Could you check a few things on this drawing? It's one solid part, dimensions in mm from its lowest x, y, z. A direction names the side the tool comes from. Give positions to 0.01 mm unless a question says otherwise; leave off trailing zeros. Loops run counter-clockwise (first coordinate to the right, second up) from the corner with the lowest first, then second, coordinate; pieces in that order, holes last. Notation, with made-up numbers: M 47,73.25 L 54,73.25 A18 ccw 54,84.25 Z; hole C -40,46.25 d5. An arc over 180 degrees is marked long. Answer as CSV lines item,"result". Start each with the question number.
Item 1: I want a section at C-C on y = 20. List the corners of the cut face in (x, z) for me (1 decimal).
Item 2: I want a section at A-A on x = 15.24. List the corners of the cut face in (y, z) for me (1 decimal).
Item 3: I want a section at B-B on x = 22. List the corners of the cut face in (y, z) for me (1 decimal).
Item 4: If we mould it in two halves opening along X, with no side actions, what happens to the marked faces 1, 2, 3 and 4? For each: released by +X, released by -X, zero draft, split by the parting line, or undercut.
Item 5: I want a section at D-D on z = 5.5. List the corners of the cut face in (x, y) for me.
Item 6: For the marked faces 5 and 6, which set-ups out of +Z, -Z, +X, -X, +Y, -Y let a thin tool reach every point of the face, with its end or its side?
Item 7: If I drill on line 1 along X through (y, z) = (14, 20); line 2 along Y through (x, z) = (5, 11.75); line 3 along X through (y, z) = (24.25, 13.5) (1 decimal), over which ranges is the centre line in solid material (lowest first)? Write a range as from..to.
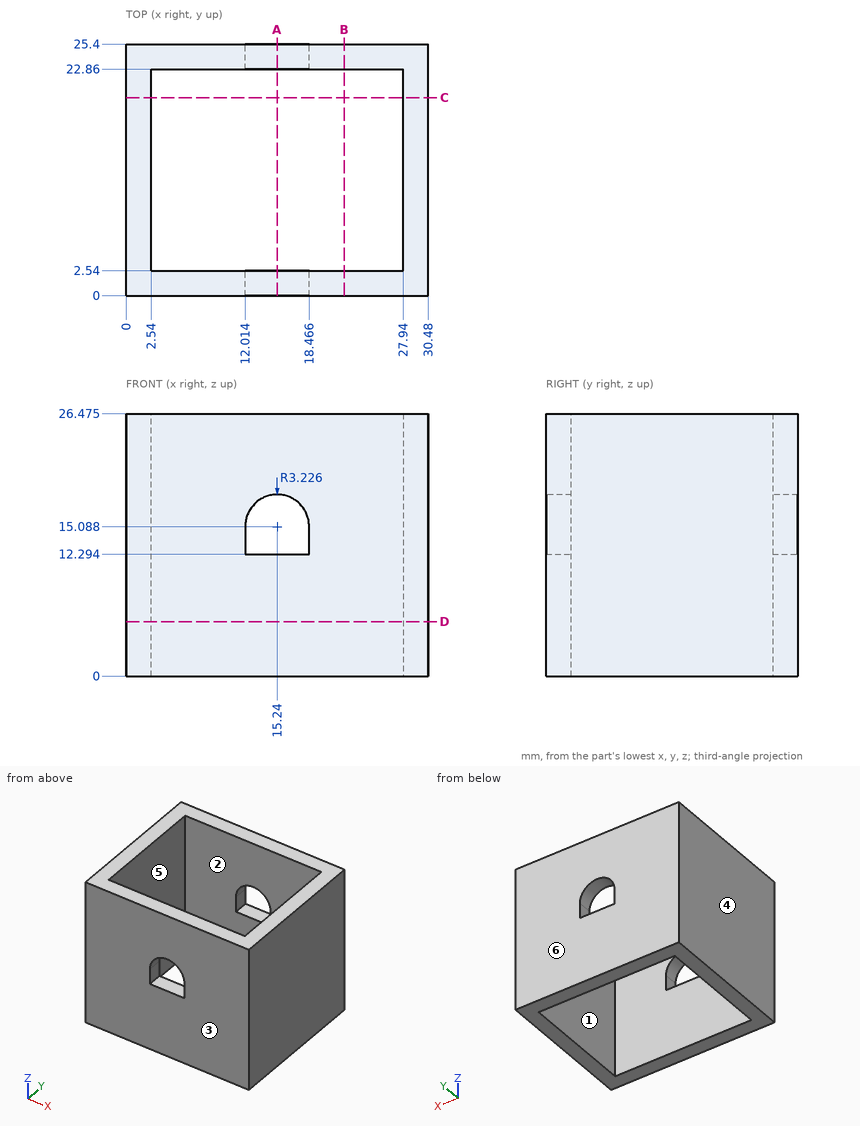
Result:
1,outline,"M 0,0 L 2.5,0 L 2.5,26.5 L 0,26.5 Z; M 27.9,0 L 30.5,0 L 30.5,26.5 L 27.9,26.5 Z"
2,outline,"M 0,0 L 2.5,0 L 2.5,12.3 L 0,12.3 Z; M 0,18.3 L 2.5,18.3 L 2.5,26.5 L 0,26.5 Z; M 22.9,0 L 25.4,0 L 25.4,12.3 L 22.9,12.3 Z; M 22.9,18.3 L 25.4,18.3 L 25.4,26.5 L 22.9,26.5 Z"
3,outline,"M 0,0 L 2.5,0 L 2.5,26.5 L 0,26.5 Z; M 22.9,0 L 25.4,0 L 25.4,26.5 L 22.9,26.5 Z"
4,face 1,"undercut"
4,face 2,"undercut"
4,face 3,"zero draft"
4,face 4,"released by -X"
5,outline,"M 0,0 L 30.48,0 L 30.48,25.4 L 0,25.4 Z; hole M 2.54,2.54 L 27.94,2.54 L 27.94,22.86 L 2.54,22.86 Z"
6,face 5,"+Z, -Z"
6,face 6,"+Z, -Z, +X, -X, +Y"
7,line 1,"0..2.54, 27.94..30.48"
7,line 2,"0..2.54, 22.86..25.4"
7,line 3,"0..12, 18.5..30.5"
